Verification items for the finished model (mm, model axes). Round coordinates to 2 decimals unless told otherwise and drop trailing zeros. Order: outer loops, then holes, each group sorted by start corner. A loop starts at its lowest first (then second) coordinate and runs counter-clockwise, first axis right, second up. Notation, with made-up numbers: M 13.5,54.25 L 38.5,54.25 A12 cw 38.5,68.25 Z; hole C -26,45.25 d3. An arc over 180 degrees is marked long. Return JSON: item names as keys, results as strings. Group by question number.
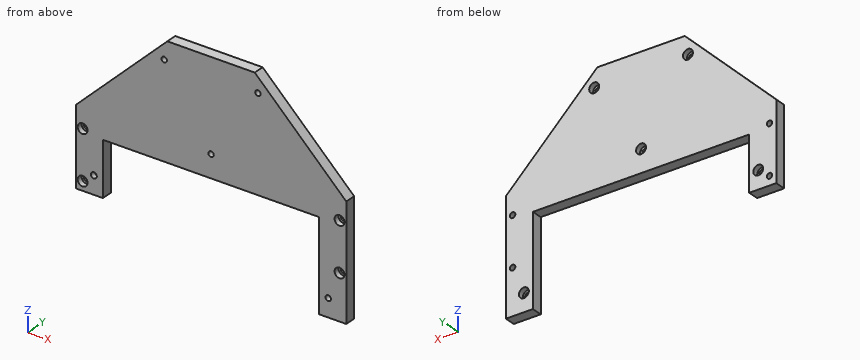
from build123d import *

# Parameters (mm, degrees)
F0_R     = 3
F0_R_2   = 3.25
F1_DEPTH = 12
F2_R     = 5.5
F3_DEPTH = 6
F4_R     = 5.5
F5_DEPTH = 6


with BuildPart() as f1:
    # F0 (on Front) → F1 (new body)
    with BuildSketch(Plane.XZ):
        Polygon((-300, -99), (-300, -185), (-270, -185), (-270, -125), (-30, -125), (-30, -225), (0, -225), (0, -99), (-101.5, 0), (-198.5, 0), align=None)
        with Locations((-292.5, -175)):
            Circle(F0_R, mode=Mode.SUBTRACT)
        with Locations((-280, -165)):
            Circle(F0_R_2, mode=Mode.SUBTRACT)
        with Locations((-292.5, -121)):
            Circle(F0_R, mode=Mode.SUBTRACT)
        with Locations((-20, -205)):
            Circle(F0_R, mode=Mode.SUBTRACT)
        with Locations((-7.5, -175)):
            Circle(F0_R, mode=Mode.SUBTRACT)
        with Locations((-7.5, -121)):
            Circle(F0_R, mode=Mode.SUBTRACT)
        with Locations((-202, -20)):
            Circle(F0_R, mode=Mode.SUBTRACT)
        with Locations((-150, -100)):
            Circle(F0_R, mode=Mode.SUBTRACT)
        with Locations((-98, -20)):
            Circle(F0_R, mode=Mode.SUBTRACT)
    extrude(amount=F1_DEPTH)

    # F2 (on face) → F3 (cut)
    with BuildSketch(Plane.XZ.offset(12)):
        with Locations((-292.5, -175)):
            Circle(F2_R)
        with Locations((-292.5, -121)):
            Circle(F2_R)
        with Locations((-7.5, -175)):
            Circle(F2_R)
        with Locations((-7.5, -121)):
            Circle(F2_R)
    extrude(amount=-F3_DEPTH, mode=Mode.SUBTRACT)

    # F4 (on face) → F5 (cut)
    with BuildSketch(Plane(origin=(0, 0, 0), x_dir=(-1, 0, 0), z_dir=(0, 1, 0))):
        with Locations((20, -205)):
            Circle(F4_R)
        with Locations((280, -165)):
            Circle(F4_R)
        with Locations((98, -20)):
            Circle(F4_R)
        with Locations((202, -20)):
            Circle(F4_R)
        with Locations((150, -100)):
            Circle(F4_R)
    extrude(amount=-F5_DEPTH, mode=Mode.SUBTRACT)


solid = f1.part
1. Thickness scan on line 1 along X through (y, z) = (-3.25, -121); line 2 along X through (y, z) = (-8.75, -152); line 3 along X through (y, z) = (-5.5, -175). Record the ranges inside material, lowest first. Write a range as from..to.
2. Cross-section at D-D (x = -280). Enter the section's corners in (y, z).
3. Go/stop test with flat-tipped pins: pin 1 (3.5 mm diameter, centred on x = -152, z = -99, fed in from +Y); pin 2 (5.5 mm diameter, centred on x = -9.5, z = -174, fed in from -Y); pin 3 (3 mm diameter, centred on x = -88.5, y = -3, fed in from -Z). Record where each tip stops, or that it passes through.
4. Cross-section at A-A (z = -139). Enter the section's corners in (x, y), plus the area to 3 significant figures.
5. Cross-section at B-B (y = -2). Give the number of separate pieces and of enclosed holes in the cut face, plus the area to 3 significant figures.
6. Cross-section at C-C (z = -165). Enter the section's corners in (x, y), plus the area to 3 significant figures.
Computed:
{
 "1": {"line 1": "x = -300..-295.5, -289.5..-10.5, -4.5..0", "line 2": "x = -300..-270, -30..0", "line 3": "x = -300..-295.5, -289.5..-270, -30..-10.5, -4.5..0"},
 "2": {"outline": "M -12,-185 L 0,-185 L 0,-170.5 L -6,-170.5 L -6,-168.25 L -12,-168.25 Z; M -12,-161.75 L -6,-161.75 L -6,-159.5 L 0,-159.5 L 0,-79.49 L -12,-79.49 Z"},
 "3": {"pin 1": "stops at y = -6", "pin 2": "stops at y = -6", "pin 3": "stops at z = -125"},
 "4": {"outline": "M -300,-12 L -270,-12 L -270,0 L -300,0 Z; M -30,-12 L 0,-12 L 0,0 L -30,0 Z", "area": "720 mm²"},
 "5": {"separate pieces": "1", "enclosed holes": "9", "area": "31,700 mm²"},
 "6": {"outline": "M -300,-12 L -283.25,-12 L -283.25,-6 L -285.5,-6 L -285.5,0 L -300,0 Z; M -276.75,-12 L -270,-12 L -270,0 L -274.5,0 L -274.5,-6 L -276.75,-6 Z; M -30,-12 L 0,-12 L 0,0 L -30,0 Z", "area": "615 mm²"}
}
